Verification items for the finished model (mm, model axes). A direction names the side the tool comes from. Give positions to 0.01 mm unless a question says otherwise; leave off trailing zeros. Write each loop counter-clockwise with the first axis right and the second up, starting at its lowest first coordinate (ties: lowest second). Pieces come first, ordered by that corner, then holes. Notation, with made-up numbers: M -18,81.5 L 3,81.5 A7 ccw 3,86.5 Z; hole C 28,-2.75 d5. An arc over 180 degrees is marked long. Write item = value, one per line.
from build123d import *

# Parameters (mm, degrees)
F0_W      = 360
F0_H      = 170
F1_DEPTH  = 180
F2_W      = 8
F2_H      = 22
F3_DEPTH  = 24
F4_R      = 4.5
F5_DEPTH  = 25
F6_R      = 4.5
F7_DEPTH  = 25
F8_W      = 12
F8_H      = 4
F9_W      = 4
F9_H      = 4
F10_DEPTH = 3


with BuildPart() as f1:
    # F0 (on Top) → F1 (new body)
    with BuildSketch(Plane.XY):
        Rectangle(F0_W, F0_H)
    extrude(amount=F1_DEPTH)

    # F2 (on face) → F3 (join)
    with BuildSketch(Plane.XY.offset(180)):
        Polygon((-100, -85), (0, -85), (100, -85), (100, -35), (135, -35), (135, 85), (0, 85), (-135, 85), (-135, -35), (-100, -35), align=None)
        with Locations((-135, -60)):
            Rectangle(F2_W, F2_H)
        with Locations((135, -60)):
            Rectangle(F2_W, F2_H)
    extrude(amount=F3_DEPTH)

    # F4 (on face) → F5 (cut)
    with BuildSketch(Plane(origin=(-139, 0, 0), x_dir=(0, -1, 0), z_dir=(-1, 0, 0))):
        with Locations((60, 192)):
            Circle(F4_R)
    extrude(amount=-F5_DEPTH, mode=Mode.SUBTRACT)

    # F6 (on face) → F7 (cut)
    with BuildSketch(Plane.YZ.offset(139)):
        with Locations((-60, 192)):
            Circle(F6_R)
    extrude(amount=-F7_DEPTH, mode=Mode.SUBTRACT)

    # F8 (on face) + F9 (on face) → F10 (cut)
    with BuildSketch(Plane.XY.offset(180)):
        with Locations((-159, -60)):
            Rectangle(F8_W, F8_H)
    with BuildSketch(Plane.XY.offset(180)):
        with Locations((155, -61.877079308)):
            Rectangle(F9_W, F9_H)
        with Locations((159, -61.877079308)):
            Rectangle(F9_W, F9_H)
        with Locations((163, -61.877079308)):
            Rectangle(F9_W, F9_H)
        with Locations((159, -57.877079308)):
            Rectangle(F9_W, F9_H)
        with Locations((159, -65.877079308)):
            Rectangle(F9_W, F9_H)
    extrude(amount=-F10_DEPTH, mode=Mode.SUBTRACT)


solid = f1.part
1) Draft check along Z on faces 4 (the flat face through (-118, -35, 192)), 5 (the cylindrical face through (-135.06, -59.02, 187.61)), 6 (the flat face through (-135, -60, 204)). Enter one of: +Z half, -Z half, draft (parallel to the pull), parting line (faces both ways), or undercut.
From the geometry:
face_4 = draft
face_5 = undercut
face_6 = +Z half
2) Cross-section at C-C on x = -122.5. Record the boundary of the cut face in (y, z), plus the area to 3 significant figures.
From the geometry:
outline = M -85,0 L 85,0 L 85,204 L -35,204 L -35,180 L -85,180 Z
area = 33,500 mm^2
3) Cross-section at A-A on z = 192. Record the boundary of the cut face in (x, y), plus the area to 3 significant figures.
From the geometry:
outline = M -139,-71 L -131,-71 L -131,-64.5 L -139,-64.5 Z; M -139,-55.5 L -131,-55.5 L -131,-49 L -139,-49 Z; M -135,-35 L -100,-35 L -100,-85 L 100,-85 L 100,-35 L 135,-35 L 135,85 L -135,85 Z; M 131,-71 L 139,-71 L 139,-64.5 L 131,-64.5 Z; M 131,-55.5 L 139,-55.5 L 139,-49 L 131,-49 Z
area = 42,600 mm^2
4) Cross-section at B-B on y = 2. Record the boundary of the cut face in (x, z).
From the geometry:
outline = M -180,0 L 180,0 L 180,180 L 135,180 L 135,204 L -135,204 L -135,180 L -180,180 Z
5) Tool access check on faces 1 (the flat face through (-100, -60, 192)), 2 (the flat face through (-135, -71, 192)), 3 (the flat face through (139, -65, 192)). Record the directions out of +Z, -Z, +X, -X, +Y, -Y that give a thin tool (end or side, any length) a straight path to the whole face; none if there is none.
From the geometry:
face_1 = +Z, -Y
face_2 = +Z, -X, -Y
face_3 = +Z, +X, +Y, -Y
6) Material ranges on probe 1 along Z at (x, y) = (137, -60); probe 2 along Z at (x, y) = (-165, 48), recorded low to high. Write a range as from..to.
From the geometry:
probe_1 = 0..187.5, 196.5..204
probe_2 = 0..180
7) Depth check by flat-ended pin: P1, Ø4, axis at x = 133, z = 193, coming from the -Y side; P2, Ø17.5, axis at y = -63.5, z = 197.5, coming from the +X side; P3, Ø24, axis at y = -60, z = 195.5, coming from the -X side. Enter the tip coordinate at first touch or a pass-through.
From the geometry:
P1 = -71
P2 = 139
P3 = -139
